```python
from build123d import *

# Parameters (mm, degrees)
SKETCH2_W          = 5
SKETCH2_H          = 2
CUT_EXTRUDE1_DEPTH = 10


with BuildPart() as part:
    # Sketch1 → Revolve1 (revolve)
    with BuildSketch(Plane.XY):
        with BuildLine():
            Line((4.5, -75.119728996), (4.5, -78.119728996))
            Line((4.5, -78.119728996), (5, -78.119728996))
            Line((5, -78.119728996), (5, -112.929313237))
            Line((5, -112.929313237), (4.5, -112.929313237))
            Line((4.5, -112.929313237), (4.5, -117.929313237))
            Line((4.5, -117.929313237), (0, -117.929313237))
            Line((0, -117.929313237), (0, -63.929313237))
            ThreePointArc((0, -63.929313237), (6.030659269, -68.004205243), (4.5, -75.119728996))
        make_face()
    revolve(axis=Axis((0, -29.874534884, 0), (0, 1, 0)))

    # Sketch2 → Cut-Extrude1 (cut)
    with BuildSketch(Plane(origin=(0, -117.929313237, 0), x_dir=(-1, 0, 0), z_dir=(0, -1, 0))):
        Rectangle(SKETCH2_W, SKETCH2_H)
    extrude(amount=-CUT_EXTRUDE1_DEPTH, mode=Mode.SUBTRACT)


solid = part.part
```
The model under review builds one solid part; all positions refer to its coordinate system, in mm. A direction names the side the tool comes from. Round coordinates to 2 decimals unless told otherwise and drop trailing zeros. Loops run counter-clockwise (first coordinate to the right, second up) from the corner with the lowest first, then second, coordinate; pieces in that order, holes last.
1) Consider section C-C on y = -90. State the section outline as (x, z) points.
Values follow:
outline: circle Ø10 at (0, 0)
2) Consider section D-D on x = -3.25. State the section outline as (y, z) points.
Values follow:
outline: (-117.93, -3.11) - (-112.93, -3.11) - (-112.93, -3.8) - (-78.12, -3.8) - (-78.12, -3.11) - (-75.12, -3.11) arc R5.63 ccw (long way) to (-75.12, 3.11) - (-78.12, 3.11) - (-78.12, 3.8) - (-112.93, 3.8) - (-112.93, 3.11) - (-117.93, 3.11) - close
3) Clearance check with flat-ended pins moving along their axes: P1, Ø1.6, axis at y = -112, z = 0.5, coming from the +X side; P2, Ø3, axis at x = -4, y = -108, coming from the -Z side; P3, Ø1, axis at y = -111, z = 0, coming from the -X side. State where each tip first meets the part, or that it passes through.
Values follow:
P1: stops at x = 5
P2: stops at z = -4.33
P3: stops at x = -5
4) Tool access review of faces 1 (the face through (0, -117.929, 2)), 2 (the face through (2.5, -113, 0)): name each direction out of +Z, -Z, +X, -X, +Y, -Y from which nothing blocks a thin tool from reaching the whole face with its end or side.
Values follow:
face 1: +Z, -Z, +X, -X, -Y
face 2: -Y
5) Wall thickness on line 1 along X through (y, z) = (-114, -0.25); line 2 along Y through (x, z) = (-4, 2.75); line 3 along Y through (x, z) = (-4, 2.5): over which ranges is each line inside the solid? List them lowest first.
Values follow:
line 1: x = -4.49 to -2.5, 2.5 to 4.49
line 2: y = -112.93 to -78.12, -74.75 to -66.11
line 3: y = -112.93 to -78.12, -74.9 to -65.96
6) The part is to be moulded in two halves that separate along Y. For faces 3 (the face through (0, -113, -1)), 4 (the face through (-0.59, -76.64, -4.46)), 5 (the face through (0, -107.929, 0)), say which applies: pulls with the +Y half, pulls with the -Y half, needs draft (parallel to the pull), parting line crosses it, or undercut.
Values follow:
face 3: needs draft
face 4: undercut
face 5: pulls with the -Y half
7) Consider section B-B on z = 0. State the section outline as (x, y) points.
Values follow:
outline: (-5, -112.93) - (-4.5, -112.93) - (-4.5, -117.93) - (-2.5, -117.93) - (-2.5, -107.93) - (2.5, -107.93) - (2.5, -117.93) - (4.5, -117.93) - (4.5, -112.93) - (5, -112.93) - (5, -78.12) - (4.5, -78.12) - (4.5, -75.12) arc R6.5 ccw (long way) to (-4.5, -75.12) - (-4.5, -78.12) - (-5, -78.12) - close
8) Consider section A-A on x = 0. State the section outline as (y, z) points.
Values follow:
outline: (-117.93, -4.5) - (-112.93, -4.5) - (-112.93, -5) - (-78.12, -5) - (-78.12, -4.5) - (-75.12, -4.5) arc R6.5 ccw (long way) to (-75.12, 4.5) - (-78.12, 4.5) - (-78.12, 5) - (-112.93, 5) - (-112.93, 4.5) - (-117.93, 4.5) - (-117.93, 1) - (-107.93, 1) - (-107.93, -1) - (-117.93, -1) - close
